from build123d import *

# Parameters (mm, degrees)
ESQUISSE1_W                    = 196.3
ESQUISSE1_H                    = 60
BOSS_EXTRU_1_DEPTH             = 2.7
ESQUISSE3_W                    = 9.8
ESQUISSE3_H                    = 2.7
ENL_V_MAT_EXTRU_1_DEPTH        = 2.7
R_P_TITION_LIN_AIRE2_COUNT     = 5
R_P_TITION_LIN_AIRE2_PITCH     = 20
R_P_TITION_LIN_AIRE2_COL_COUNT = 6
R_P_TITION_LIN_AIRE2_COL_PITCH = 20
ESQUISSE5_R                    = 2.1
ENL_V_MAT_EXTRU_3_DEPTH        = 10


with BuildPart() as part:
    # Esquisse1 → Boss.-Extru.1 (new body)
    with BuildSketch(Plane.XY):
        with Locations((0, -30)):
            Rectangle(ESQUISSE1_W, ESQUISSE1_H)
    extrude(amount=BOSS_EXTRU_1_DEPTH)

    # Esquisse3 → Enl_v. mat.-Extru.1 (cut)
    with BuildSketch(Plane.XY):
        with Locations((10, -58.65)):
            Rectangle(ESQUISSE3_W, ESQUISSE3_H)
    enl_v_mat_extru_1 = extrude(amount=ENL_V_MAT_EXTRU_1_DEPTH, mode=Mode.SUBTRACT)

    # R_p_tition lin_aire2: Enl_v. mat.-Extru.1 ×5
    with Locations(*[(i * R_P_TITION_LIN_AIRE2_PITCH, 0, 0) for i in range(1, R_P_TITION_LIN_AIRE2_COUNT)]):
        add(enl_v_mat_extru_1, mode=Mode.SUBTRACT)

    # R_p_tition lin_aire2 col: Enl_v. mat.-Extru.1 ×6
    with Locations(*[(-i * R_P_TITION_LIN_AIRE2_COL_PITCH, 0, 0) for i in range(1, R_P_TITION_LIN_AIRE2_COL_COUNT)]):
        add(enl_v_mat_extru_1, mode=Mode.SUBTRACT)

    # Esquisse5 → Enl_v. mat.-Extru.3 (cut)
    with BuildSketch(Plane.XY):
        with Locations(Location((-83.081, -30, 0), (0, 0, 180))):
            Circle(ESQUISSE5_R)
        with Locations(Location((-1.081, -30, 0), (0, 0, 180))):
            Circle(ESQUISSE5_R)
        with Locations(Location((80.919, -30, 0), (0, 0, 180))):
            Circle(ESQUISSE5_R)
    extrude(amount=ENL_V_MAT_EXTRU_3_DEPTH, mode=Mode.SUBTRACT)


solid = part.part
Work out the finished part from the listing and answer in its coordinate system (mm). Give positions to 0.01 mm unless a question says otherwise; leave off trailing zeros. Loops run counter-clockwise (first coordinate to the right, second up) from the corner with the lowest first, then second, coordinate; pieces in that order, holes last. Notation, with made-up numbers: (-10, -40) -> (33, -40) arc R23 cw to (33, -28) -> close; hole circle Ø6 at (58, 6.5). An arc over 180 degrees is marked (long way). Use a Markdown table: item, result. Add a question column.
1. Section B-B on z = 1.05 is taken. State how many separate pieces and enclosed holes the cut face has, and give its area (3 significant figures).
2. Section C-C on x = 33 is taken. Determine the outline of the cut face in (y, z), and give its area (3 significant figures).
3. Determine the mould class of faces 1 (the flat face through (-1, -23, 2.7)), 2 (the cylindrical face through (83.017, -30.092, 1.331)) for opening direction X: released by +X, released by -X, zero draft, split by the parting line, or undercut.
4. A flat-ended cylindrical pin translates along its axis: pin 1 Ø0.8 at (x, z) = (10.5, 1) entering from -Y. Find the tip coordinate at first contact, or state that the pin passes through.
5. Find the intervals of material crossed by probe 1 along X at (y, z) = (-30, 1.8); probe 2 along Y at (x, z) = (82, 1.2); probe 3 along Y at (x, z) = (-27.5, 0.55), in increasing order.
6. Section A-A on y = -30 is taken. Determine the outline of the cut face in (x, z).
Results below:
| question | item | result |
|---|---|---|
| 1 | separate pieces | 1 |
| 1 | enclosed holes | 3 |
| 1 | area | 11,500 mm^2 |
| 2 | outline | (-57.3, 0) -> (0, 0) -> (0, 2.7) -> (-57.3, 2.7) -> close |
| 2 | area | 155 mm^2 |
| 3 | face 1 | zero draft |
| 3 | face 2 | undercut |
| 4 | pin 1 | stops at y = -57.3 |
| 5 | probe 1 | x = -98.15 to -85.18, -80.98 to -3.18, 1.02 to 78.82, 83.02 to 98.15 |
| 5 | probe 2 | y = -60 to -31.8, -28.2 to 0 |
| 5 | probe 3 | y = -57.3 to 0 |
| 6 | outline | (-98.15, 0) -> (-85.18, 0) -> (-85.18, 2.7) -> (-98.15, 2.7) -> close; (-80.98, 0) -> (-3.18, 0) -> (-3.18, 2.7) -> (-80.98, 2.7) -> close; (1.02, 0) -> (78.82, 0) -> (78.82, 2.7) -> (1.02, 2.7) -> close; (83.02, 0) -> (98.15, 0) -> (98.15, 2.7) -> (83.02, 2.7) -> close |
